from build123d import *

# Parameters (mm, degrees)
ESBO_O4_R                = 3.5
ESBO_O4_R_2              = 1.5
RESSALTO_EXTRUS_O1_DEPTH = 3


with BuildPart() as part:
    # Esboço4 → Ressalto-extrusão1 (new body)
    with BuildSketch(Plane(origin=(0, 0, 0), x_dir=(1, 0, 0), z_dir=(0, 1, 0))):
        with BuildLine():
            Line((0, 100), (10, 100))
            ThreePointArc((10, 100), (15.870896117, 57.454662802), (16.6322809, 14.512918173))
            ThreePointArc((16.6322809, 14.512918173), (16.571046781, 8.001087588), (16.933775774, 1.499079062))
            ThreePointArc((16.933775774, 1.499079062), (0, -17), (-16.933775774, 1.499079062))
            ThreePointArc((-16.933775774, 1.499079062), (-16.571046781, 8.001087588), (-16.6322809, 14.512918173))
            ThreePointArc((-16.6322809, 14.512918173), (-15.870896117, 57.454662802), (-10, 100))
            Line((-10, 100), (0, 100))
        make_face()
        with Locations(Location((0, 0, 0), (0, 0, 270))):
            Circle(ESBO_O4_R, mode=Mode.SUBTRACT)
        with Locations(Location((9.2, 82.966613318, 0), (0, 0, 270))):
            Circle(ESBO_O4_R_2, mode=Mode.SUBTRACT)
        with Locations(Location((-9.2, 82.966613318, 0), (0, 0, 90))):
            Circle(ESBO_O4_R_2, mode=Mode.SUBTRACT)
        Polygon((6.2, 94.466613318), (6.2, 71.466613318), (-6.2, 71.466613318), (-6.2, 94.466613318), (-2.5, 94.466613318), (-2.5, 96.466613318), (2.5, 96.466613318), (2.5, 94.466613318), align=None, mode=Mode.SUBTRACT)
        Polygon((0, -15), (-0.5, -15), (-0.5, -9), (0.5, -9), (0.5, -15), align=None, mode=Mode.SUBTRACT)
        Polygon((0.5, 15), (0, 15), (-0.5, 15), (-0.5, 9), (0.5, 9), align=None, mode=Mode.SUBTRACT)
    extrude(amount=RESSALTO_EXTRUS_O1_DEPTH)


solid = part.part
Geometry: final body of the model. Coordinates: model frame, mm. A direction names the side the tool comes from. Coordinates: 2 decimals unless noted, no trailing zeros. Order: outer loops, then holes, each group sorted by start corner. A loop starts at its lowest first (then second) coordinate and runs counter-clockwise, first axis right, second up.
(1) Access query for faces 4 (the face through (0, 0, -29)), 5 (the face through (15.824, 1.479, -58.054)), 6 (the face through (-16.573, 1.479, -7.91)), 7 (the face through (-4, 1, -94.467)). Directions: +Z, -Z, +X, -X, +Y, -Y. A direction counts if a zero-diameter tool reaches every point of the face in a straight line with its end or side. Return the directions, or none.
(2) Section query D-D (z = 4.5). Return the cut outline in (x, y), plus the area to 3 significant figures.
(3) Section query C-C (z = -55). Return the cut outline in (x, y).
(4) Material intervals for probe 1 along X at (y, z) = (1.65, 0); probe 2 along X at (y, z) = (0.45, -82); probe 3 along Z at (x, y) = (-5.5, 0.5), sorted ascending.
(5) Section query A-A (z = -85.5). Return the cut outline in (x, y).
(6) First-contact query: pin 1 (1.5 mm diameter, centred on x = -12.5, z = -66.5, fed in from -Y); pin 2 (0.9 mm diameter, centred on y = 1, z = -85, fed in from +X); pin 3 (1 mm diameter, centred on x = 1, y = 0.5, fed in from +Z); pin 4 (1.5 mm diameter, centred on x = 3.5, y = 1.5, fed in from +Z). Flat tips, straight axial feed; report the tip coordinate or a pass-through.
(7) Draft query along Z for faces 1 (the face through (-8.287, 1.479, -81.776)), 2 (the face through (0, 1, -100)), 3 (the face through (0, 3, -29)). Return one class per face: pulls with the +Z half, pulls with the -Z half, needs draft (parallel to the pull), parting line crosses it, or undercut.
(8) Section query B-B (y = 1.4). Return the cut outline in (x, z), plus the area to 3 significant figures.
Solution:
1. face 4: +Z, -Z, +X, -X, -Y
1. face 5: +X, +Y, -Y
1. face 6: -X, +Y, -Y
1. face 7: +Y, -Y
2. outline: (-16.39, 0) - (16.39, 0) - (16.39, 3) - (-16.39, 3) - close
2. area: 98.4 mm2
3. outline: (-16.05, 0) - (16.05, 0) - (16.05, 3) - (-16.05, 3) - close
4. probe 1: x = -17 to -3.5, 3.5 to 17
4. probe 2: x = -13.12 to -10.35, -8.05 to -6.2, 6.2 to 8.05, 10.35 to 13.12
4. probe 3: z = -100 to -94.47, -71.47 to 16.09
5. outline: (-12.58, 0) - (-6.2, 0) - (-6.2, 3) - (-12.58, 3) - close; (6.2, 0) - (12.58, 0) - (12.58, 3) - (6.2, 3) - close
6. pin 1: stops at y = 0
6. pin 2: stops at x = 12.73
6. pin 3: stops at z = 16.99
6. pin 4: stops at z = 16.78
7. face 1: undercut
7. face 2: pulls with the -Z half
7. face 3: needs draft
8. outline: (-16.93, -1.5) arc R100 cw to (-16.63, -14.51) arc R359.93 ccw to (-10, -100) - (10, -100) arc R359.93 ccw to (16.63, -14.51) arc R100 cw to (16.93, -1.5) arc R17 ccw (long way) to start; hole circle Ø3 at (-9.2, -82.97); hole (-6.2, -94.47) - (-2.5, -94.47) - (-2.5, -96.47) - (2.5, -96.47) - (2.5, -94.47) - (6.2, -94.47) - (6.2, -71.47) - (-6.2, -71.47) - close; hole circle Ø7 at (0, 0); hole (-0.5, -15) - (0.5, -15) - (0.5, -9) - (-0.5, -9) - close; hole (-0.5, 9) - (0.5, 9) - (0.5, 15) - (-0.5, 15) - close; hole circle Ø3 at (9.2, -82.97)
8. area: 3,150 mm2
